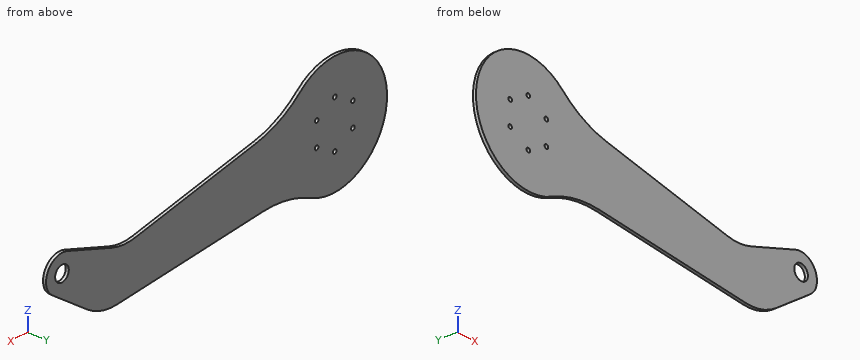
```python
from build123d import *

# Parameters (mm, degrees)
SKETCH1_R           = 2
SKETCH1_R_2         = 7.5
BOSS_EXTRUDE2_DEPTH = 3
FILLET1_R           = 50
FILLET2_R           = 100


with BuildPart() as part:
    # Sketch1 → Boss-Extrude2 (new body)
    with BuildSketch(Plane(origin=(0, 0, 0), x_dir=(1, 0, 0), z_dir=(0, 1, 0))):
        with BuildLine():
            Line((257.543524338, 52.623283), (43.136797408, 38.01929391))
            ThreePointArc((43.136797408, 38.01929391), (-57.072915612, -6.99516287), (51.041719813, -26.476269347))
            Line((51.041719813, -26.476269347), (232.634460204, 5.800541986))
            Line((232.634460204, 5.800541986), (294.037229007, -16.452822314))
            ThreePointArc((294.037229007, -16.452822314), (315.449808374, -8.21908883), (310.311776158, 14.139210461))
            Line((310.311776158, 14.139210461), (257.543524338, 52.623283))
        make_face()
        with Locations(Location((19.918584287, 11.5, 0), (0, 0, 270))):
            Circle(SKETCH1_R, mode=Mode.SUBTRACT)
        with Locations(Location((-19.918584287, 11.5, 0), (0, 0, 270))):
            Circle(SKETCH1_R, mode=Mode.SUBTRACT)
        with Locations(Location((0, 23, 0), (0, 0, 270))):
            Circle(SKETCH1_R, mode=Mode.SUBTRACT)
        with Locations(Location((0, -23, 0), (0, 0, 270))):
            Circle(SKETCH1_R, mode=Mode.SUBTRACT)
        with Locations(Location((-19.918584287, -11.5, 0), (0, 0, 270))):
            Circle(SKETCH1_R, mode=Mode.SUBTRACT)
        with Locations(Location((19.918584287, -11.5, 0), (0, 0, 270))):
            Circle(SKETCH1_R, mode=Mode.SUBTRACT)
        with Locations(Location((300, 0, 0), (0, 0, 270))):
            Circle(SKETCH1_R_2, mode=Mode.SUBTRACT)
    extrude(amount=BOSS_EXTRUDE2_DEPTH)

    # Fillet1
    fillet1_edges = [part.edges().sort_by_distance(p)[0] for p in [
        (232.634460204, 1.5, -5.800541986),
        (257.543524338, 1.5, -52.623283),
    ]]
    fillet(fillet1_edges, radius=FILLET1_R)

    # Fillet2
    fillet2_edges = [part.edges().sort_by_distance(p)[0] for p in [
        (51.041719813, 1.5, 26.476269347),
        (43.136797408, 1.5, -38.01929391),
    ]]
    fillet(fillet2_edges, radius=FILLET2_R)


solid = part.part
```
For this review, take the finished solid that the model builds, in its own axes (mm). Coordinates: 2 decimals unless noted, no trailing zeros. Order: outer loops, then holes, each group sorted by start corner. A loop starts at its lowest first (then second) coordinate and runs counter-clockwise, first axis right, second up. Notation, with made-up numbers: (15, 86) -> (56, 86) arc R24 ccw to (56, 102) -> close; hole circle Ø1 at (-16.5, 89.5). An arc over 180 degrees is marked (long way). Answer as CSV lines item,"result".
Q1. Clearance check with a flat-ended pin moving along its axis: pin 1 Ø1 at (y, z) = (1, 3.5) entering from +X. State where the tip first meets the part, or that it passes through.
Model answer:
pin 1,"stops at x = 317.24"
Q2. We need section C-C (x = 210.5). State the section outline as (y, z) points, plus the area to 3 significant figures.
Model answer:
outline,"(0, -49.42) -> (3, -49.42) -> (3, -1.87) -> (0, -1.87) -> close"
area,"143 mm2"
Q3. We need section A-A (x = 300). State the section outline as (y, z) points, plus the area to 3 significant figures.
Model answer:
outline,"(0, -21.66) -> (3, -21.66) -> (3, -7.5) -> (0, -7.5) -> close; (0, 7.5) -> (3, 7.5) -> (3, 17.5) -> (0, 17.5) -> close"
area,"72.5 mm2"
Q4. We need section B-B (y = 1.6). State the section outline as (x, z) points (3 decimals).
Model answer:
outline,"(26.199, -51.184) arc R100 cw to (78.559, -40.432) -> (239.387, -51.387) arc R50 ccw to (272.247, -41.9) -> (310.312, -14.139) arc R17.5 ccw to (294.037, 16.453) -> (245.23, -1.236) arc R50 cw to (219.444, -3.456) -> (85.998, 20.263) arc R100 cw to (37.785, 43.342) arc R57.5 ccw (long way) to start; hole circle Ø4 at (-19.919, -11.5); hole circle Ø4 at (-19.919, 11.5); hole circle Ø4 at (0, -23); hole circle Ø4 at (0, 23); hole circle Ø4 at (19.919, -11.5); hole circle Ø4 at (19.919, 11.5); hole circle Ø15 at (300, 0)"
Q5. We need section D-D (x = 99.5). State the section outline as (y, z) points.
Model answer:
outline,"(0, -41.86) -> (3, -41.86) -> (3, 17.86) -> (0, 17.86) -> close"
Q6. Wall thickness on line 1 along X through (y, z) = (1.9, -11.5); line 2 along Z through (x, y) = (87.5, 2); line 3 along Z through (x, y) = (172.5, 1.45): over which ranges is each line inside the solid? List them lowest first. Write a range as [from, to].
Model answer:
line 1,"x = [-56.34, -21.92], [-17.92, 17.92], [21.92, 313.19]"
line 2,"z = [-41.04, 20]"
line 3,"z = [-46.83, 4.89]"
